Geometry: final body of the model. Coordinates: model frame, mm. A direction names the side the tool comes from. Round coordinates to 2 decimals unless told otherwise and drop trailing zeros. Loops run counter-clockwise (first coordinate to the right, second up) from the corner with the lowest first, then second, coordinate; pieces in that order, holes last. Notation, with made-up numbers: (89.5, 23) - (120.5, 23) arc R31 cw to (120.5, 60) - close; hole circle Ø7 at (49.5, 41.25). An arc over 180 degrees is marked (long way). Return JSON: item names as keys, results as strings. Group by question number.
1. First-contact query: pin 1 Ø5 at (x, z) = (116.5, 1238) entering from -Y; pin 2 Ø6 at (y, z) = (373, 1265.5) entering from +X; pin 3 Ø1.5 at (x, z) = (90, 470) entering from +Y. Flat tips, straight axial feed; report the tip coordinate or a pass-through.
2. Draft query along Y for faces 3 (the face through (61.21, 459.945, 811.2)), 4 (the face through (-465, 25, 1600)), 5 (the face through (20.844, 469.538, 788.8)). Return one class per face: +Y half, -Y half, draft (parallel to the pull), parting line (faces both ways), or undercut.
3. Section A-A on x = 0. Return loops of the section in (y, z).
4. Section C-C on z = 1450. Return loops of the section in (x, y).
5. Section D-D on x = -188.5. Return loops of the section in (y, z).
6. Material intervals for probe 1 along Z at (x, y) = (0, -464.25); probe 2 along X at (y, z) = (-4.5, 225); probe 3 along X at (y, z) = (-30.5, 1126), sorted ascending.
7. Section B-B on y = -168.5. Return loops of the section in (x, z).
8. Set-up query: faces 1 (the face through (17.535, -466.274, 186.287)), 2 (the face through (-465, 25, 0)). Return all of +Z, -Z, +X, -X, +Y, -Y with unobstructed straight access to the full face (end or side cutting, diameter ignored); none if empty.
Autodesk Inventor part; units mm, degrees
ref_plane "SHELL Plane" through (-332.3402, -332.3402, 0) normal (0.7071, -0.7071, 0) x (0.7071, 0.7071, 0)
ref_plane "ACCESS Plane" through (-213, -870, 0) normal (0, -1, 0) x (1, 0, 0)
ref_plane "OUTER Plane" through (-38, -670, 0) normal (0, -1, 0) x (1, 0, 0)
sketch "floor angle sketch" plane through (0, 0, 0) normal (0, 0, 1) x (1, 0, 0)
  line L0 (0, 0) -> (0, -240.1382) construction
  line L1 (0, 0) -> (0, -870)
  line L2 (-332.3402, -332.3402) -> (332.3402, 332.3402) construction
  circle A0 centre (0, 0) radius 470 construction
  line L3 (0, 0) -> (0, -670)
  line L4 (-38, -670) -> (38, -670)
  line L5 (-213, -870) -> (213, -870)
  line L6 (0, 0) -> (-263.3555, -723.5633)
  line L7 (0, 0) -> (0, -570)
  line L8 (-38, -570) -> (38, -570)
  line L9 (-324.4355, -701.332) -> (-202.2755, -745.7946)
  dimension "d51" = 940
  dimension "d52" = 45
  dimension "d54" = 0
  dimension "d55" = 0
  dimension "d56" = 426
  dimension "d58" = 76
  dimension "d59" = 76
  dimension "d60" = 0
  dimension "d61" = 570
  dimension "d62" = 130
  dimension "d63" = 20
  dimension "d64" = 670
  dimension "d65" = 770
  dimension "d66" = 870
ref_plane "SHELL Plane" through (-332.3402, -332.3402, 0) normal (0.7071, -0.7071, 0) x (0.7071, 0.7071, 0)
ref_plane "ACCESS Plane" through (-213, -870, 0) normal (0, -1, 0) x (1, 0, 0)
ref_plane "OUTER Plane" through (-38, -670, 0) normal (0, -1, 0) x (1, 0, 0)
ref_plane "INNER Plane" through (-38, -570, 0) normal (0, -1, 0) x (1, 0, 0)
ref_plane "CHARGE Plane" through (-324.4355, -701.332, 0) normal (-0.342, -0.9397, 0) x (0.9397, -0.342, 0)
sketch "Sketch13" plane through (-332.3402, -332.3402, 0) normal (0.7071, -0.7071, 0) x (0.7071, 0.7071, 0)
  line L0 (470, 0) -> (470, 892.6829)
  line L1 (0, 0) -> (6, 0)
  line L2 (6, 0) -> (6, 1600)
  line L3 (6, 1600) -> (0, 1600)
  line L4 (0, 1600) -> (0, 0)
  dimension "d75" = 1600
  dimension "d76" = 6
  dimension "d77" = 940
revolve "Revolution2" add sketch "Sketch13" angle 359.9 about axis through (0, 0, 0) along (0, 0, 1)
sketch "Sketch14" plane through (-213, -870, 0) normal (0, -1, 0) x (1, 0, 0)
  circle A0 centre (213, 1060) radius 213
  line L0 (683, 1600) -> (-257, 1600)
  point P0 (213, 0)
  point P1 (-119.3402, 1600)
  point P2 (-119.9197, 1600)
  dimension "d80" = 426
  dimension "d93" = 540
extrude "ACCESS" cut sketch "Sketch14" against normal up to next
sketch "Sketch15" plane through (-38, -570, 0) normal (0, -1, 0) x (1, 0, 0)
  circle A0 centre (38, 220) radius 38
  point P0 (38, 0)
  dimension "d84" = 76
  dimension "d85" = 220
extrude "INNER" cut sketch "Sketch15" against normal up to next
sketch "Sketch16" plane through (-38, -670, 0) normal (0, -1, 0) x (1, 0, 0)
  circle A0 centre (38, 1450) radius 38
  line L0 (508, 1600) -> (-432, 1600)
  point P0 (38, 0)
  point P1 (-294.3402, 1600)
  point P2 (-294.9197, 1600)
  dimension "d89" = 76
  dimension "d92" = 150
extrude "Extrusion9" cut sketch "Sketch16" against normal up to next
equation "\"BendRadius\" = Thickness"
equation "\"BendReliefWidth\" = Thickness"
equation "\"BendReliefDepth\" = 0.5 * Thickness"
equation "\"CornerReliefSize\" = 4 * Thickness"
equation "\"MinimumRemnant\" = 2 * Thickness"
equation "\"TransitionRadius\" = BendRadius"
equation "\"JacobiRadiusSize\" = BendRadius"
equation "\"GapSize\" = Thickness"
properties part number "TZS 0902 SHELL" material "Steel"
Taken from the geometry:
{
 "1": {"pin 1": "y = -455.83", "pin 2": "x = 289.83", "pin 3": "y = 461.45"},
 "2": {"face 3": "undercut", "face 4": "draft", "face 5": "parting line"},
 "3": {"outline": "(-470, 0) - (-464, 0) - (-464, 182) - (-470, 182) - close; (-470, 258) - (-464, 258) - (-464, 847) - (-470, 847) - close; (-470, 1273) - (-464, 1273) - (-464, 1412) - (-470, 1412) - close; (-470, 1488) - (-464, 1488) - (-464, 1600) - (-470, 1600) - close; (464, 0) - (470, 0) - (470, 1600) - (464, 1600) - close"},
 "4": {"outline": "(-332.92, -331.76) - (-328.67, -327.52) arc R464 cw (long way) to (38, -462.44) - (38, -468.46) arc R470 ccw (long way) to start; (-332.34, -332.34) arc R470 ccw to (-38, -468.46) - (-38, -462.44) arc R464 cw to (-328.1, -328.1) - close"},
 "5": {"outline": "(-430.54, 0) - (-423.99, 0) - (-423.99, 960.82) - (-430.54, 960.82) - close; (-430.54, 1159.18) - (-423.99, 1159.18) - (-423.99, 1600) - (-430.54, 1600) - close; (423.99, 0) - (430.54, 0) - (430.54, 1600) - (423.99, 1600) - close"},
 "6": {"probe 1": "0 to 182, 258 to 847, 1273 to 1412, 1488 to 1600", "probe 2": "-469.98 to -463.98, 463.98 to 469.98", "probe 3": "-469.01 to -463, 463 to 469.01"},
 "7": {"outline": "(-438.76, 0) - (-432.32, 0) - (-432.32, 1600) - (-438.76, 1600) - close; (432.32, 0) - (438.76, 0) - (438.76, 1600) - (432.32, 1600) - close"},
 "8": {"face 1": "-Y", "face 2": "-Z, +X, -X, +Y, -Y"}
}
